from build123d import *

# Parameters (mm, degrees)
SZKIC1_W                    = 32
SZKIC1_H                    = 32
DODANIE_WYCI_GNI_CIE2_DEPTH = 1
SZKIC3_W                    = 30
SZKIC3_H                    = 28
DODANIE_WYCI_GNI_CIE3_DEPTH = 1
SZKIC2_W                    = 30
SZKIC2_H                    = 1.1
DODANIE_WYCI_GNI_CIE4_DEPTH = 10
ZAOKR_GLENIE1_R             = 0.1
ZAOKR_GLENIE3_R             = 0.5
ZAOKR_GLENIE4_R             = 0.3
WYTNIJ_WYCI_GNI_CIE1_DEPTH  = 2


with BuildPart() as part:
    # Szkic1 → Dodanie-wyciągnięcie2 (new body)
    with BuildSketch(Plane(origin=(0, 0, 0), x_dir=(1, 0, 0), z_dir=(0, 1, 0))):
        Rectangle(SZKIC1_W, SZKIC1_H)
        with BuildLine():
            Line((-14.495689014, 19.445436483), (19.445436483, -14.495689014))
            ThreePointArc((19.445436483, -14.495689014), (19.445436483, -19.445436483), (14.495689014, -19.445436483))
            Line((14.495689014, -19.445436483), (-19.445436483, 14.495689014))
            ThreePointArc((-19.445436483, 14.495689014), (-19.445436483, 19.445436483), (-14.495689014, 19.445436483))
        make_face()
    extrude(amount=DODANIE_WYCI_GNI_CIE2_DEPTH)

    # Szkic3 → Dodanie-wyciągnięcie3 (add)
    with BuildSketch(Plane(origin=(0, 1, 0), x_dir=(1, 0, 0), z_dir=(0, 1, 0))):
        Rectangle(SZKIC3_W, SZKIC3_H)
    extrude(amount=DODANIE_WYCI_GNI_CIE3_DEPTH)

    # Szkic2 → Dodanie-wyciągnięcie4 (add)
    with BuildSketch(Plane(origin=(0, 1, 0), x_dir=(1, 0, 0), z_dir=(0, 1, 0))):
        with Locations((0, 13.45)):
            Rectangle(SZKIC2_W, SZKIC2_H)
        with Locations((0, 11.208333333)):
            Rectangle(SZKIC2_W, SZKIC2_H)
        with Locations((0, 8.966666667)):
            Rectangle(SZKIC2_W, SZKIC2_H)
        with Locations((0, 6.725)):
            Rectangle(SZKIC2_W, SZKIC2_H)
        with Locations((0, 4.483333333)):
            Rectangle(SZKIC2_W, SZKIC2_H)
        with Locations((0, 2.241666667)):
            Rectangle(SZKIC2_W, SZKIC2_H)
        Rectangle(SZKIC2_W, SZKIC2_H)
        with Locations((0, -2.241666667)):
            Rectangle(SZKIC2_W, SZKIC2_H)
        with Locations((0, -4.483333333)):
            Rectangle(SZKIC2_W, SZKIC2_H)
        with Locations((0, -6.725)):
            Rectangle(SZKIC2_W, SZKIC2_H)
        with Locations((0, -8.966666667)):
            Rectangle(SZKIC2_W, SZKIC2_H)
        with Locations((0, -11.208333333)):
            Rectangle(SZKIC2_W, SZKIC2_H)
        with Locations((0, -13.45)):
            Rectangle(SZKIC2_W, SZKIC2_H)
    extrude(amount=DODANIE_WYCI_GNI_CIE4_DEPTH)

    # Zaokrąglenie1
    zaokr_glenie1_edges = [part.edges().sort_by_distance(p)[0] for p in [
        (-15, 1, 0),
        (0, 1, 14),
        (15, 1, 0),
        (0, 1, -14),
    ]]
    fillet(zaokr_glenie1_edges, radius=ZAOKR_GLENIE1_R)

    # Zaokrąglenie3
    zaokr_glenie3_edges = [part.edges().sort_by_distance(p)[0] for p in [
        (0, 2, -6.175),
        (0, 2, -7.275),
        (0, 2, -3.933333333),
        (0, 2, -5.033333333),
        (0, 2, -1.691666667),
        (0, 2, -2.791666667),
        (0, 2, 0.55),
        (0, 2, -0.55),
        (0, 2, 2.791666667),
        (0, 2, 1.691666667),
        (0, 2, 5.033333333),
        (0, 2, 3.933333333),
        (0, 2, 7.275),
        (0, 2, 6.175),
        (0, 2, 9.516666667),
        (0, 2, 8.416666667),
        (0, 2, 11.758333333),
        (0, 2, 10.658333333),
        (0, 2, 12.9),
        (0, 2, -12.9),
        (0, 2, -10.658333333),
        (0, 2, -11.758333333),
        (0, 2, -8.416666667),
        (0, 2, -9.516666667),
    ]]
    fillet(zaokr_glenie3_edges, radius=ZAOKR_GLENIE3_R)

    # Zaokrąglenie4
    zaokr_glenie4_edges = [part.edges().sort_by_distance(p)[0] for p in [
        (0, 11, -6.175),
        (0, 11, -7.275),
        (0, 11, -3.933333333),
        (0, 11, -5.033333333),
        (0, 11, -1.691666667),
        (0, 11, -2.791666667),
        (0, 11, 0.55),
        (0, 11, -0.55),
        (0, 11, 2.791666667),
        (0, 11, 1.691666667),
        (0, 11, 5.033333333),
        (0, 11, 3.933333333),
        (0, 11, 7.275),
        (0, 11, 6.175),
        (0, 11, 9.516666667),
        (0, 11, 8.416666667),
        (0, 11, 11.758333333),
        (0, 11, 10.658333333),
        (0, 11, 14),
        (0, 11, 12.9),
        (0, 11, -12.9),
        (0, 11, -14),
        (0, 11, -10.658333333),
        (0, 11, -11.758333333),
        (0, 11, -8.416666667),
        (0, 11, -9.516666667),
    ]]
    fillet(zaokr_glenie4_edges, radius=ZAOKR_GLENIE4_R)

    # Szkic4 → Wytnij-wyciągnięcie1 (cut, through all)
    with BuildSketch(Plane(origin=(0, 1, 0), x_dir=(1, 0, 0), z_dir=(0, 1, 0))):
        with BuildLine():
            Line((-15.909902577, 18.03122292), (-14.439120472, 16.560440815))
            ThreePointArc((-14.439120472, 16.560440815), (-14.439120472, 14.439120472), (-16.560440815, 14.439120472))
            Line((-16.560440815, 14.439120472), (-18.03122292, 15.909902577))
            ThreePointArc((-18.03122292, 15.909902577), (-18.03122292, 18.03122292), (-15.909902577, 18.03122292))
        make_face()
        with BuildLine():
            Line((15.909902577, -18.03122292), (14.439120472, -16.560440815))
            ThreePointArc((14.439120472, -16.560440815), (14.439120472, -14.439120472), (16.560440815, -14.439120472))
            Line((16.560440815, -14.439120472), (18.03122292, -15.909902577))
            ThreePointArc((18.03122292, -15.909902577), (18.03122292, -18.03122292), (15.909902577, -18.03122292))
        make_face()
    extrude(amount=-WYTNIJ_WYCI_GNI_CIE1_DEPTH, mode=Mode.SUBTRACT)


solid = part.part
Design review of the part built by this model. Coordinates are the model's own, in mm. A direction names the side the tool comes from. Give positions to 0.01 mm unless a question says otherwise; leave off trailing zeros. Write item = value, one per line.
Q1. To check wall thickness, follow line 1 (X direction, y = 1.25, z = -7); line 2 (Y direction, x = 3, z = -15.5); line 3 (Y direction, x = 13, z = 8). State the ranges of each line that lie inside material, in increasing order. Write a range as [from, to].
Output values:
line_1 = [-15, 15]
line_2 = [0, 1]
line_3 = [0, 2.01]
Q2. We need section A-A (y = 4.5). Count the separate pieces of the cut face and the enclosed holes in it, plus the area to 3 significant figures.
Output values:
separate_pieces = 13
enclosed_holes = 0
area = 429 mm^2
Q3. Draft analysis for pull direction X (two halves, no side actions). For faces 1 (the flat face through (12.8, 0.49, 17.75)), 2 (the flat face through (0, 7, -11.758)), 3 (the flat face through (15.185, 0.507, 17.306)), 4 (the cylindrical face through (18.05, 0.51, 18.01)), state which applies: +X half, -X half, draft (parallel to the pull), parting line (faces both ways), or undercut.
Output values:
face_1 = -X half
face_2 = draft
face_3 = undercut
face_4 = undercut
Q4. For faces 5 (the flat face through (0, 6, -14)), 6 (the flat face through (-15, 5, 0)), 7 (the flat face through (0, 7, 12.9)), list the 3-axis set-ups (+Z, -Z, +X, -X, +Y, -Y) from which the entire face can be reached by the end or side of a thin tool; tool diameter is ignored.
Output values:
face_5 = -Z, +X, -X, +Y
face_6 = +Z, -Z, -X, +Y
face_7 = +X, -X, +Y
Q5. Insertion check: pin 1 (6.5 mm diameter, centred on x = 5.5, y = 8, fed in from -Z); pin 2 (0.5 mm diameter, centred on y = 0.5, z = 7.5, fed in from -X); pin 3 (2.5 mm diameter, centred on x = 3, y = 8, fed in from +Z). Each pin has a flat end and moves straight along its axis. Give the tip position at first contact, or say it passes through.
Output values:
pin_1 = -14
pin_2 = -16
pin_3 = 14
